```python
from build123d import *

# Parameters (mm, degrees)
F0_W     = 10
F0_H     = 12
F1_DEPTH = 26
F2_R     = 0.762
F3_R     = 1.5
F4_DEPTH = 10
F5_R     = 0.79375
F6_DEPTH = 3.175


with BuildPart() as f1:
    # F0 (on Top) → F1 (new body)
    with BuildSketch(Plane.XY):
        Rectangle(F0_W, F0_H)
    extrude(amount=F1_DEPTH)

    # F2
    f2_edges = [f1.edges().sort_by_distance(p)[0] for p in [
        (-5, -6, 13),
        (-5, 6, 13),
        (5, -6, 13),
        (5, 6, 13),
    ]]
    fillet(f2_edges, radius=F2_R)

    # F3 (on face) → F4 (join)
    with BuildSketch(Plane.XY.offset(26)):
        Circle(F3_R)
    extrude(amount=F4_DEPTH)

    # F5 (on face) → F6 (cut)
    with BuildSketch(Plane.XY.offset(26)):
        with Locations((0, 4.015625)):
            Circle(F5_R)
        with Locations((0, -4.015625)):
            Circle(F5_R)
    extrude(amount=-F6_DEPTH, mode=Mode.SUBTRACT)


solid = f1.part
```
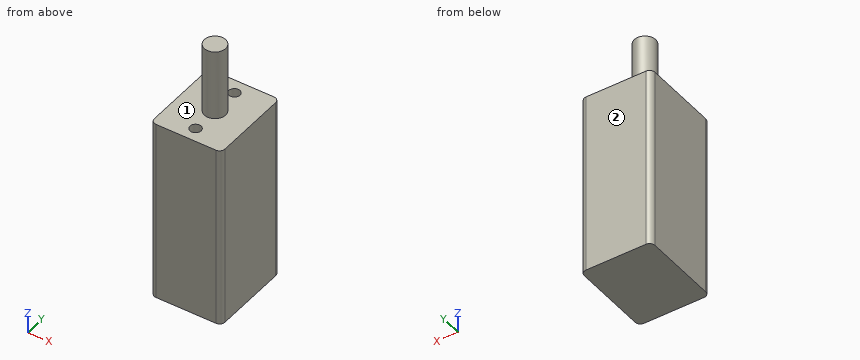
Design review of the part built by this model. Coordinates are the model's own, in mm. Face numbers are marked on the shaded views. A direction names the side the tool comes from. Give positions to 0.01 mm unless a question says otherwise; leave off trailing zeros. Order: outer loops, then holes, each group sorted by start corner. A loop starts at its lowest first (then second) coordinate and runs counter-clockwise, first axis right, second up. Notation, with made-up numbers: (39, -13.75) -> (53, -13.75) arc R23 cw to (53, 19.25) -> close; hole circle Ø10 at (60, 10). An arc over 180 degrees is marked (long way). Write item = value, one per line. Start each with the question number.
(1) We need section B-B on y = 0. Write out the cut boundary in (x, z).
(2) For pin 1 (2.5 mm diameter, centred on x = 0, y = 4.02, fed in from +Z); pin 2 (1.3 mm diameter, centred on x = 0, y = -4.02, fed in from +Z) (3 decimals), all flat-tipped, find the tip position at first contact; note any pin that passes through.
(3) We need section A-A on x = 0. Write out the cut boundary in (y, z) (3 decimals).
(4) To check wall thickness, follow line 1 along Y through (x, z) = (0, 24.25); line 2 along Z through (x, y) = (2.5, -0.5); line 3 along Y through (x, z) = (-4.5, 10.5). State the ranges of each line that lie inside material, in increasing order.
(5) We need section C-C on z = 23.5. Write out the cut boundary in (x, y).
(6) For the marked faces 1 and 2, list the 3-axis set-ups (+Z, -Z, +X, -X, +Y, -Y) from which the entire face can be reached by the end or side of a thin tool; tool diameter is ignored.
Numbers:
q1.outline = (-5, 0) -> (5, 0) -> (5, 26) -> (1.5, 26) -> (1.5, 36) -> (-1.5, 36) -> (-1.5, 26) -> (-5, 26) -> close
q2.pin_1 = 26
q2.pin_2 = 22.825
q3.outline = (-6, 0) -> (6, 0) -> (6, 26) -> (4.809, 26) -> (4.809, 22.825) -> (3.222, 22.825) -> (3.222, 26) -> (1.5, 26) -> (1.5, 36) -> (-1.5, 36) -> (-1.5, 26) -> (-3.222, 26) -> (-3.222, 22.825) -> (-4.809, 22.825) -> (-4.809, 26) -> (-6, 26) -> close
q4.line_1 = -6 to -4.81, -3.22 to 3.22, 4.81 to 6
q4.line_2 = 0 to 26
q4.line_3 = -5.95 to 5.95
q5.outline = (-5, -5.24) arc R0.76 ccw to (-4.24, -6) -> (4.24, -6) arc R0.76 ccw to (5, -5.24) -> (5, 5.24) arc R0.76 ccw to (4.24, 6) -> (-4.24, 6) arc R0.76 ccw to (-5, 5.24) -> close; hole circle Ø1.59 at (0, -4.02); hole circle Ø1.59 at (0, 4.02)
q6.face_1 = +Z
q6.face_2 = +Z, -Z, +X, -X, +Y
